Input: part model. Units: mm. Frame: model coordinates. A direction names the side the tool comes from. Coordinates: 2 decimals unless noted, no trailing zeros. Order: outer loops, then holes, each group sorted by start corner. A loop starts at its lowest first (then second) coordinate and runs counter-clockwise, first axis right, second up. Notation, with made-up numbers: (54.5, -9.75) -> (89.5, -9.75) arc R30 ccw to (89.5, 23.25) -> close; hole circle Ø6 at (50, 64). An arc over 180 degrees is marked (long way). Answer as CSV lines item,"result".
Autodesk Inventor part; units mm, degrees
ref_plane "YZ Plane" through (0, 0, 0) normal (1, 0, 0) x (0, 1, 0)
ref_plane "XZ Plane" through (0, 0, 0) normal (0, 1, 0) x (-1, 0, 0)
ref_plane "XY Plane" through (0, 0, 0) normal (0, 0, 1) x (1, 0, 0)
sketch "スケッチ2" plane through (0, 0, 0) normal (0, 1, 0) x (-1, 0, 0)
  line L0 (19, 24) -> (45, 24)
  line L1 (45, 24) -> (45, 0)
  line L2 (45, 0) -> (19, 0)
  line L3 (19, 0) -> (19, 24)
  circle A0 centre (32, 24) radius 6.25
  line L4 (19, 24) -> (45, 24)
  line L5 (45, 24) -> (45, 27)
  line L6 (45, 27) -> (19, 27)
  line L7 (19, 27) -> (19, 24)
  line L8 (-45, 24) -> (-19, 24)
  line L9 (-19, 24) -> (-19, 0)
  line L10 (-19, 0) -> (-45, 0)
  line L11 (-45, 0) -> (-45, 24)
  circle A1 centre (-32, 24) radius 6.25
  line L12 (-45, 24) -> (-19, 24)
  line L13 (-19, 24) -> (-19, 27)
  line L14 (-19, 27) -> (-45, 27)
  line L15 (-45, 27) -> (-45, 24)
  line L16 (0, -6.05) -> (0, 36.3)
  line L17 (64.3086, 0) -> (-70.8513, 0)
  line L18 (-19, 9) -> (19, 9)
  line L19 (19, 9) -> (19, 0)
  line L20 (19, 0) -> (-19, 0)
  line L21 (-19, 0) -> (-19, 9)
  point P0 (0, 0)
  point P1 (-51.5428, 0.5174)
  point P2 (19, 0)
  point P3 (37.4829, 27)
  point P4 (26.5171, 27)
  point P5 (-26.5171, 27)
  point P6 (-37.4829, 27)
  point P7 (-19, 0)
  dimension "d4" = 26
  dimension "d5" = 24
  dimension "d6" = 12.5
  dimension "d7" = 3
  dimension "d8" = 26
  dimension "d9" = 24
  dimension "d10" = 12.5
  dimension "d11" = 3
  dimension "d12" = 64
  dimension "d13" = 9
extrude "プレート2" add sketch "スケッチ2" along normal blind 1.5 contours A0 L6 L5 L0 | L0 L1 L2 L3 A0 | L0 L7 L6 A0 | L17 L16 L18 L3 | L17 L9 L18 L16 | L10 L11 L8 A1 L9 | L8 A1 L14 L13 | L15 L14 A1 L8
sketch "スケッチ3" plane through (0, 1.5, 0) normal (0, 1, 0) x (1, 0, 0)
  line L0 (45, 0) -> (45, -27)
  line L1 (19, -27) -> (19, -9)
  line L2 (-42.5, -3) -> (-21.5, -3)
  line L3 (-21.5, -3) -> (-21.5, -17.75)
  line L4 (-21.5, -17.75) -> (-42.5, -17.75)
  line L5 (-42.5, -17.75) -> (-42.5, -3)
  line L6 (21.5, -3) -> (42.5, -3)
  line L7 (42.5, -3) -> (42.5, -17.75)
  line L8 (42.5, -17.75) -> (21.5, -17.75)
  line L9 (21.5, -17.75) -> (21.5, -3)
  arc A0 (-26.5171, -27) -> (-37.4829, -27) centre (-32, -24) ccw
  line L10 (-42.5, -6) -> (-21.5, -6)
  line L11 (-21.5, -6) -> (-21.5, -14.75)
  line L12 (-21.5, -14.75) -> (-42.5, -14.75)
  line L13 (-42.5, -14.75) -> (-42.5, -6)
  line L14 (21.5, -6) -> (42.5, -6)
  line L15 (42.5, -6) -> (42.5, -14.75)
  line L16 (42.5, -14.75) -> (21.5, -14.75)
  line L17 (21.5, -14.75) -> (21.5, -6)
  circle A1 centre (-42.5, -24) radius 0.85
  circle A2 centre (-42.5, -3) radius 0.85
  circle A3 centre (-21.5, -3) radius 0.85
  circle A4 centre (-21.5, -24) radius 0.85
  circle A5 centre (21.5, -24) radius 0.85
  circle A6 centre (42.5, -24) radius 0.85
  circle A7 centre (42.5, -3) radius 0.85
  circle A8 centre (21.5, -3) radius 0.85
  circle A9 centre (7, -5.5) radius 0.8
  circle A10 centre (-7, -5.5) radius 0.8
  arc A11 (37.4829, -27) -> (26.5171, -27) centre (32, -24) ccw
  arc A12 (37.4829, -27) -> (26.5171, -27) centre (32, -24) ccw
  line L18 (45, -27) -> (37.4829, -27)
  line L19 (-45, 0) -> (45, 0)
  line L20 (-45, -27) -> (-45, 0)
  line L21 (-37.4829, -27) -> (-45, -27)
  arc A13 (-26.5171, -27) -> (-37.4829, -27) centre (-32, -24) ccw
  line L22 (-19, -27) -> (-26.5171, -27)
  line L23 (-19, -9) -> (-19, -27)
  line L24 (19, -9) -> (-19, -9)
  line L25 (26.5171, -27) -> (19, -27)
  point P0 (0, 0)
  dimension "d20" = 3
  dimension "d21" = 3
extrude "切り取り1" cut sketch "スケッチ3" against normal blind 1.5 contours L16 L9 L14 L7 | L12 L5 L10 L3 | A7 L6 L7 | L7 L6 A7 | A8 L6 L9 | L9 L6 A8 | A3 L2 L3 | L3 L2 A3 | A2 L2 L5 | L5 L2 A2 | A1 | A4 | A5 | A6 | A9 | A10
fillet "フィレット1" radius 3 20 edges at (-21.5, 0.75, 6) (-21.5, 0.75, 14.75) (-42.5, 0.75, 14.75) (-42.5, 0.75, 6) (-37.4829, 0.75, 27) (-45, 0.75, 27) (-26.5171, 0.75, 27) (-19, 0.75, 27) (19, 0.75, 27) (26.5171, 0.75, 27) (37.4829, 0.75, 27) (45, 0.75, 27) (45, 0.75, 0) (-45, 0.75, 0) (-19, 0.75, 9) (19, 0.75, 9) (42.5, 0.75, 14.75) (21.5, 0.75, 14.75) (21.5, 0.75, 6) (42.5, 0.75, 6)
equation "\"d11\" = d7"
equation "\"d18\" = Thickness"
equation "\"d14\" = Thickness"
equation "\"BendRadius\" = Thickness"
equation "\"BendReliefWidth\" = Thickness"
equation "\"BendReliefDepth\" = 0.5 * Thickness"
equation "\"CornerReliefSize\" = 4 * Thickness"
equation "\"MinimumRemnant\" = 2 * Thickness"
equation "\"TransitionRadius\" = BendRadius"
equation "\"JacobiRadiusSize\" = BendRadius"
equation "\"GapSize\" = Thickness"
properties part number "hipjoint_upper"
1. Reachability of faces 4 (the face through (-42.5, 1, 10)), 5 (the face through (-44.14, 0.76, 26.1)), 6 (the face through (-19, 1, 18)) from +Z, -Z, +X, -X, +Y, -Y: full face, straight path, thin tool, end or side. Return the list, or none.
Findings:
face 4,"+Y, -Y"
face 5,"+Z, -X, +Y, -Y"
face 6,"+Z, +Y, -Y"
2. Ray query, line 1 along X through (y, z) = (0.6, 3); line 2 along X through (y, z) = (1.45, 5.25); line 3 along X through (y, z) = (1.2, 12). Return the intervals inside material, ascending.
Findings:
line 1,"x = -45 to -43.35, -41.65 to -22.35, -20.65 to 20.65, 22.35 to 41.65, 43.35 to 45"
line 2,"x = -45 to -7.76, -6.24 to 6.24, 7.76 to 45"
line 3,"x = -45 to -42.49, -21.51 to -19, 19 to 21.51, 42.49 to 45"
3. Contact query for a flat-ended pin moving along its axis: pin 1 (1.5 mm diameter, centred on x = -42.5, z = 24, fed in from -Y). Output: stop coordinate, or through.
Findings:
pin 1,"passes through"
4. Cut plane C-C (y = 0.9). State how many separate pieces and enclosed holes the cut face has, plus the area to 3 significant figures.
Findings:
separate pieces,"1"
enclosed holes,"12"
area,"1,160 mm2"
5. Cut plane D-D (x = -30). Return the cut outline in (y, z), plus the area to 3 significant figures.
Findings:
outline,"(0, 0) -> (1.5, 0) -> (1.5, 6) -> (0, 6) -> close; (0, 14.75) -> (1.5, 14.75) -> (1.5, 18.08) -> (0, 18.08) -> close"
area,"14.0 mm2"
6. Mould query, pull axis Z, two halves, no side actions, for faces 1 (the face through (0, 1, 9)), 2 (the face through (45, 1, 13)), 3 (the face through (21.5, 1, 10)). Classes: released by +Z, released by -Z, zero draft, split by the parting line, or undercut.
Findings:
face 1,"released by +Z"
face 2,"zero draft"
face 3,"undercut"
7. Cut plane A-A (x = 32). Return the cut outline in (y, z), plus the area to 3 significant figures.
Findings:
outline,"(0, 0) -> (1.5, 0) -> (1.5, 6) -> (0, 6) -> close; (0, 14.75) -> (1.5, 14.75) -> (1.5, 17.75) -> (0, 17.75) -> close"
area,"13.5 mm2"
8. Cut plane B-B (z = 21.5). Return the cut outline in (x, y).
Findings:
outline,"(-45, 0) -> (-37.73, 0) -> (-37.73, 1.5) -> (-45, 1.5) -> close; (-26.27, 0) -> (-19, 0) -> (-19, 1.5) -> (-26.27, 1.5) -> close; (19, 0) -> (26.27, 0) -> (26.27, 1.5) -> (19, 1.5) -> close; (37.73, 0) -> (45, 0) -> (45, 1.5) -> (37.73, 1.5) -> close"
